from build123d import *

# Parameters (mm, degrees)
F0_R     = 11.2
F1_DEPTH = 7


with BuildPart() as f1:
    # F0 (on Top) → F1 (new body)
    with BuildSketch(Plane.XY):
        with BuildLine():
            ThreePointArc((-13.165616, 0.952129), (0.476375, 13.191401), (13.2, 0))
            ThreePointArc((13.2, 0), (0.476375, -13.191401), (-13.165616, -0.952129))
            Line((-13.165616, -0.952129), (-13.165616, -30.748123))
            ThreePointArc((-13.165616, -30.748123), (-0.386904, -44.739478), (13.21028, -31.542127))
            Line((13.21028, -31.542127), (13.194472, 31.165589))
            Line((13.194472, 31.165589), (13.194278, 31.936201))
            ThreePointArc((13.194278, 31.936201), (0.282113, 44.744554), (-13.165616, 32.499698))
            Line((-13.165616, 32.499698), (-13.165616, 30.59544))
            Line((-13.165616, 30.59544), (-13.165616, 0.952129))
        make_face()
        with Locations((0.010281, -31.545455)):
            Circle(F0_R, mode=Mode.SUBTRACT)
        with Locations((0, 31.547569)):
            Circle(F0_R, mode=Mode.SUBTRACT)
    extrude(amount=F1_DEPTH)


solid = f1.part
Design review of the part built by this model. Coordinates are the model's own, in mm. Coordinates: 2 decimals unless noted, no trailing zeros. Write each loop counter-clockwise with the first axis right and the second up, starting at its lowest first coordinate (ties: lowest second). Pieces come first, ordered by that corner, then holes. Notation, with made-up numbers: (3, 7) - (23, 7) arc R19 ccw to (23, 34) - close; hole circle Ø3 at (36.25, 58). An arc over 180 degrees is marked (long way). One line per item, written item: value.
1) Add section C-C (z = 2.75). State the section outline as (x, y) points.
Answer sheet:
outline: (-13.17, -30.75) arc R13.2 ccw (long way) to (13.21, -31.54) - (13.19, 31.17) - (13.19, 31.94) arc R13.2 ccw to (-13.17, 32.5) - (-13.17, 0.95) arc R13.2 cw (long way) to (-13.17, -0.95) - close; hole circle Ø22.4 at (0, 31.55); hole circle Ø22.4 at (0.01, -31.55)
2) To check wall thickness, follow probe 1 along Y at (x, z) = (0, 5); probe 2 along X at (y, z) = (-32, 1.25); probe 3 along Y at (x, z) = (-6, 3.25). State the ranges of each line that lie inside material, in increasing order.
Answer sheet:
probe 1: y = -44.75 to -42.75, -20.35 to -13.2, 13.2 to 20.35, 42.75 to 44.75
probe 2: x = -13.18 to -11.18, 11.2 to 13.2
probe 3: y = -43.3 to -41, -22.09 to -11.76, 11.76 to 22.09, 41 to 43.31
3) Mouldability with a two-part tool opening along X and no side actions: class faces 1 (the face through (-2.428, 20.614, 3.451)), 2 (the face through (-13.166, -16, 3)), 3 (the face through (-0.683, -44.727, 3.451)), 4 (the face through (6.03, -22.1, 3.45)) as +X half, -X half, draft (parallel to the pull), parting line (faces both ways), or undercut.
Answer sheet:
face 1: undercut
face 2: -X half
face 3: parting line
face 4: undercut
4) Add section D-D (x = -9.25). State the section outline as (y, z) points, plus the area to 3 significant figures.
Answer sheet:
outline: (-40.95, 0) - (-37.85, 0) - (-37.85, 7) - (-40.95, 7) - close; (-25.25, 0) - (-9.42, 0) - (-9.42, 7) - (-25.25, 7) - close; (9.42, 0) - (25.23, 0) - (25.23, 7) - (9.42, 7) - close; (37.86, 0) - (40.96, 0) - (40.96, 7) - (37.86, 7) - close
area: 265 mm2
5) Insertion check: pin 1 (2 mm diameter, centred on y = -21, z = 4, fed in from -X); pin 2 (12 mm diameter, centred on x = 4.5, y = 25, fed in from +Z); pin 3 (1.5 mm diameter, centred on y = 12.5, z = 4.5, fed in from +X). Each pin has a flat end and moves straight along its axis. Give the tip position at first contact, or say it passes through.
Answer sheet:
pin 1: stops at x = -13.17
pin 2: stops at z = 7
pin 3: stops at x = 13.2
6) Add section B-B (y = 6.5). State the section outline as (x, z) points, plus the area to 3 significant figures.
Answer sheet:
outline: (-13.17, 0) - (-11.49, 0) - (-11.49, 7) - (-13.17, 7) - close; (11.49, 0) - (13.2, 0) - (13.2, 7) - (11.49, 7) - close
area: 23.7 mm2
7) Add section A-A (x = 0). State the section outline as (y, z) points, plus the area to 3 significant figures.
Answer sheet:
outline: (-44.75, 0) - (-42.75, 0) - (-42.75, 7) - (-44.75, 7) - close; (-20.35, 0) - (-13.2, 0) - (-13.2, 7) - (-20.35, 7) - close; (13.2, 0) - (20.35, 0) - (20.35, 7) - (13.2, 7) - close; (42.75, 0) - (44.75, 0) - (44.75, 7) - (42.75, 7) - close
area: 128 mm2
